from build123d import *

# Parameters (mm, degrees)
STOCK_A_0101_1_DEPTH    = 19.05
CUT_EXTRUDE1_DEPTH      = 38.1
CUT_EXTRUDE1_DEPTH_BACK = 38.1
SKETCH1_R               = 31.115


# Read off the part's stored shape, not the designer's step: Stock-A-0101-1
with BuildPart() as part:
    # Stock-A-0101-1 outline → Stock-A-0101-1 (new body)
    with BuildSketch(Plane(origin=(0, 0, 0), x_dir=(1, 0, 0), z_dir=(0, 1, 0))):
        with BuildLine():
            Line((86.721024484, 86.721024484), (44.901280605, 44.901280605))
            ThreePointArc((44.901280605, 44.901280605), (44.901280605, -44.901280605), (-44.901280605, -44.901280605))
            Line((-44.901280605, -44.901280605), (-86.721024484, -86.721024484))
            Line((-86.721024484, -86.721024484), (-50.8, -122.642048969))
            Line((-50.8, -122.642048969), (50.8, -122.642048969))
            Line((50.8, -122.642048969), (122.642048969, -50.8))
            Line((122.642048969, -50.8), (122.642048969, 50.8))
            Line((122.642048969, 50.8), (86.721024484, 86.721024484))
        make_face()
    extrude(amount=STOCK_A_0101_1_DEPTH)

    # Sketch1 → Cut-Extrude1 (cut, two sides: drawn at the far end of the back side and taken through both)
    with BuildSketch(Plane(origin=(0, 0, 0), x_dir=(-0.7071067811865475, 0, -0.7071067811865477), z_dir=(0.7071067811865477, 0, -0.7071067811865475)).offset(-CUT_EXTRUDE1_DEPTH_BACK)):
        with Locations((-88.352048969, 41.91)):
            Circle(SKETCH1_R)
    extrude(amount=CUT_EXTRUDE1_DEPTH + CUT_EXTRUDE1_DEPTH_BACK, mode=Mode.SUBTRACT)


solid = part.part
Read the model definition and answer for the solid it produces. Units are mm, in the model's axes. A direction names the side the tool comes from. Give positions to 0.01 mm unless a question says otherwise; leave off trailing zeros. Write each loop counter-clockwise with the first axis right and the second up, starting at its lowest first coordinate (ties: lowest second). Pieces come first, ordered by that corner, then holes. Notation, with made-up numbers: (-20, 26.5) - (12, 26.5) arc R14 cw to (12, 52.5) - close; hole circle Ø7 at (-38.5, 32.5). An arc over 180 degrees is marked (long way). Return JSON: item names as keys, results as strings.
Q1. Given P1, Ø5, axis at y = 12, z = -36.5, coming from the -X side; P2, Ø10, axis at x = -14, y = 7, coming from the -Z side; P3, Ø2, axis at x = 54, y = 13.5, coming from the +Z side, each flat-ended and moving along its own axis, determine where each tip first touches the part or whether it passes through.
Reply:
{"P1": "x = 50.11", "P2": "z = 60.59", "P3": "z = 120.44"}
Q2. Consider line 1 along X through (y, z) = (18, 52); line 2 along X through (y, z) = (15.25, -38.5); line 3 along Z through (x, y) = (80.5, 16.25). Determine where each line is inside the solid, lowest interval first. Write a range as [from, to].
Reply:
{"line 1": "[-52, -36.45], [36.45, 44.79], [101.11, 121.44]", "line 2": "[50.5, 122.64]", "line 3": "[-80.5, 26.62], [69.34, 92.94]"}
Q3. For faces 4 (the face through (35.74, 15.9, 89.62)), 5 (the face through (-66, 9, 66)), determine the directions among +Z, -Z, +X, -X, +Y, -Y from which every point of the face is accessible in a straight line to the end or side of a thin tool.
Reply:
{"face 4": "+Y", "face 5": "-Z, -X, +Y, -Y"}
Q4. A cutting plane is placed at B-B, the plane x = 0. Determine the outline of the cut face in (y, z), and give its area (3 significant figures).
Reply:
{"outline": "(0, 63.5) - (19.05, 63.5) - (19.05, 122.64) - (0, 122.64) - close", "area": "1,130 mm²"}
Q5. For a pull along X with two mould halves and no side action, classify faces 1 (the face through (86.22, 9.39, 87.22)), 2 (the face through (17, 19.05, 64)), 3 (the face through (45.88, 9.39, 43.9)) as released by +X, released by -X, zero draft, split by the parting line, or undercut.
Reply:
{"face 1": "released by +X", "face 2": "zero draft", "face 3": "undercut"}
Q6. A cutting plane is placed at A-A, the plane z = 0. Determine the outline of the cut face in (x, y), and give its area (3 significant figures).
Reply:
{"outline": "(63.5, 0) - (122.64, 0) - (122.64, 19.05) - (63.5, 19.05) - close", "area": "1,130 mm²"}
